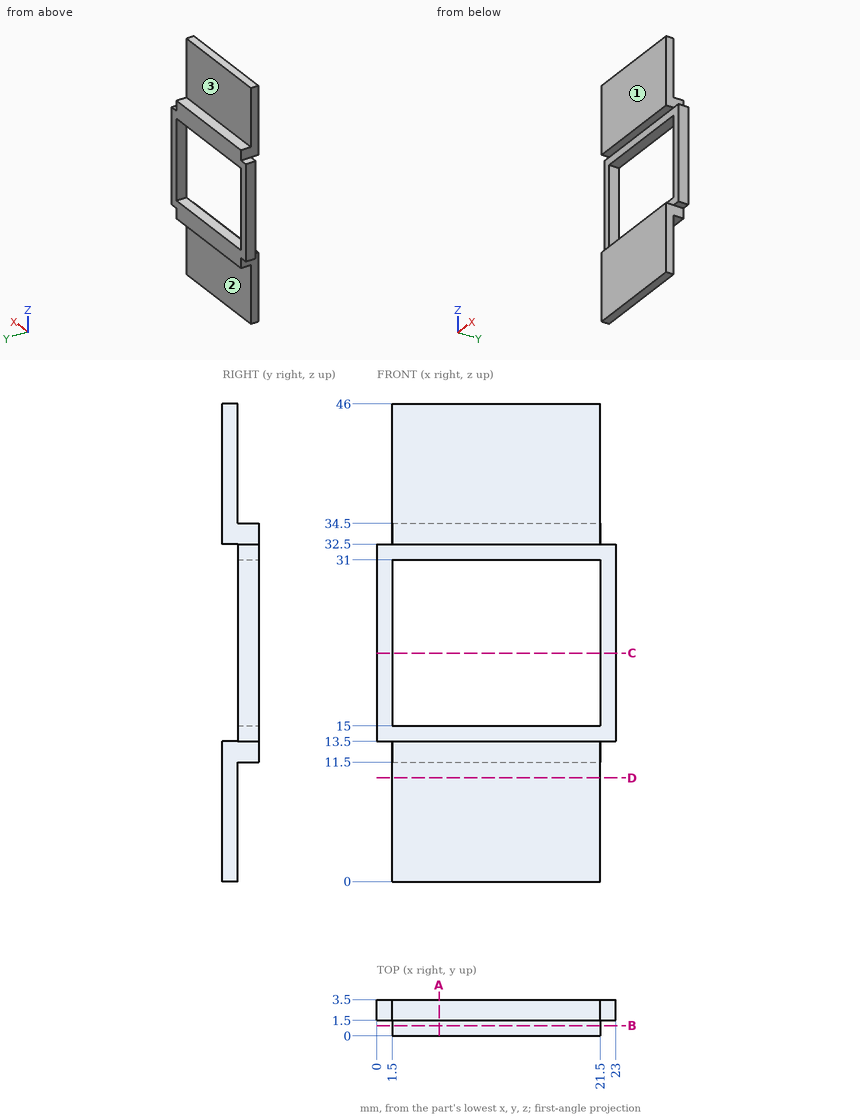
Check sheet for the drawn part. Datum: minimum x, y, z corner. Units: mm. A direction names the side the tool comes from. Round coordinates to 2 decimals unless told otherwise and drop trailing zeros. Write each loop counter-clockwise with the first axis right and the second up, starting at its lowest first coordinate (ties: lowest second). Pieces come first, ordered by that corner, then holes. Notation, with made-up numbers: (50, 79) - (89, 79) arc R28 cw to (89, 118) - close; hole circle Ø6 at (-8.5, 31.25). An arc over 180 degrees is marked (long way). Write each question's results on one line, items separated by ' | '.
(1) Sectioned sample at B-B, the plane y = 1. Enter the section's corners in (x, z).
Computed:
outline: (1.5, 0) - (21.5, 0) - (21.5, 13.5) - (1.5, 13.5) - close; (1.5, 32.5) - (21.5, 32.5) - (21.5, 46) - (1.5, 46) - close
(2) Depth check by flat-ended pin: pin 1 Ø9.5 at (x, z) = (15, 19.5) entering from -Y; pin 2 Ø1.5 at (y, z) = (3, 40.5) entering from +X; pin 3 Ø1.5 at (x, y) = (11.5, 3) entering from -Z; pin 4 Ø0.8 at (x, y) = (22.5, 2.5) entering from +Z. Enter the tip coordinate at first touch or a pass-through.
Computed:
pin 1: stops at y = 1.5 | pin 2: passes through | pin 3: stops at z = 11.5 | pin 4: stops at z = 32.5
(3) Sectioned sample at C-C, the plane z = 22. Enter the section's corners in (x, y), plus the area to 3 significant figures.
Computed:
outline: (0, 1.5) - (1.5, 1.5) - (1.5, 3.5) - (0, 3.5) - close; (21.5, 1.5) - (23, 1.5) - (23, 3.5) - (21.5, 3.5) - close | area: 6.00 mm^2
(4) Set-up check for the marked faces 1, 2 and 3: record each of +Z, -Z, +X, -X, +Y, -Y from which the full face is reachable in a straight line by a thin tool's end or side.
Computed:
face 1: +Z, -Z, +X, -X, -Y | face 2: -Z, +X, -X, +Y | face 3: +Z, +X, -X, +Y
(5) Thickness scan on probe 1 along Z at (x, y) = (11.75, 1.6); probe 2 along Z at (x, y) = (20.5, 0.5); probe 3 along X at (y, z) = (2.2, 17.5). Record the ranges inside material, lowest first. Write a range as from..to.
Computed:
probe 1: z = 11.5..15, 31..34.5 | probe 2: z = 0..13.5, 32.5..46 | probe 3: x = 0..1.5, 21.5..23
(6) Sectioned sample at D-D, the plane z = 10. Enter the section's corners in (x, y).
Computed:
outline: (1.5, 0) - (21.5, 0) - (21.5, 1.5) - (1.5, 1.5) - close
(7) Sectioned sample at A-A, the plane x = 6. Enter the section's corners in (y, z), plus the area to 3 significant figures.
Computed:
outline: (0, 0) - (1.5, 0) - (1.5, 11.5) - (3.5, 11.5) - (3.5, 15) - (1.5, 15) - (1.5, 13.5) - (0, 13.5) - close; (0, 32.5) - (1.5, 32.5) - (1.5, 31) - (3.5, 31) - (3.5, 34.5) - (1.5, 34.5) - (1.5, 46) - (0, 46) - close | area: 54.5 mm^2
